```python
from build123d import *

# Parameters (mm, degrees)
ESQUISSE1_W       = 5.08
ESQUISSE1_H       = 2.54
EXTRUSION1_DEPTH  = 4
ESQUISSE2_R       = 0.915
EXTRUSION2_DEPTH  = 0.4
ESQUISSE3_R       = 0.535
EXTRUSION3_DEPTH  = 1.065
D_ME1_FACE_RADIUS = 0.535
D_ME1_HEIGHT      = 0.535
D_ME2_FACE_RADIUS = 0.535
D_ME2_HEIGHT      = 0.535


with BuildPart() as part:
    # Esquisse1 → Extrusion1 (new body)
    with BuildSketch(Plane.XY):
        with Locations((2.54, 1.27)):
            Rectangle(ESQUISSE1_W, ESQUISSE1_H)
    extrude(amount=EXTRUSION1_DEPTH)

    # Esquisse2 → Extrusion2 (add)
    with BuildSketch(Plane.XY.offset(4)):
        with Locations(Location((3.81, 1.27, 0), (0, 0, 180))):
            Circle(ESQUISSE2_R)
        with Locations(Location((1.27, 1.27, 0), (0, 0, 180))):
            Circle(ESQUISSE2_R)
    extrude(amount=EXTRUSION2_DEPTH)

    # Esquisse3 → Extrusion3 (add)
    with BuildSketch(Plane(origin=(0, 0, 0), x_dir=(-1, 0, 0), z_dir=(0, 0, -1))):
        with Locations((-3.81, 1.27)):
            Circle(ESQUISSE3_R)
        with Locations((-1.27, 1.27)):
            Circle(ESQUISSE3_R)
    extrude(amount=EXTRUSION3_DEPTH)

    # Dôme1: a dome of height H over a round flat face of radius A is a cap of a sphere of radius (A * A + H * H) / (2 * H)
    d_me1_r = (D_ME1_FACE_RADIUS * D_ME1_FACE_RADIUS + D_ME1_HEIGHT * D_ME1_HEIGHT) / (2 * D_ME1_HEIGHT)
    d_me1_base = Plane((3.81, 1.27, -1.065), z_dir=(0, 0, -1))
    with Locations(d_me1_base.offset(D_ME1_HEIGHT - d_me1_r)):
        d_me1_ball = Sphere(d_me1_r, mode=Mode.PRIVATE)
    add(split(d_me1_ball, bisect_by=d_me1_base, keep=Keep.TOP, mode=Mode.PRIVATE))

    # Dôme2: a dome of height H over a round flat face of radius A is a cap of a sphere of radius (A * A + H * H) / (2 * H)
    d_me2_r = (D_ME2_FACE_RADIUS * D_ME2_FACE_RADIUS + D_ME2_HEIGHT * D_ME2_HEIGHT) / (2 * D_ME2_HEIGHT)
    d_me2_base = Plane((1.27, 1.27, -1.065), z_dir=(0, 0, -1))
    with Locations(d_me2_base.offset(D_ME2_HEIGHT - d_me2_r)):
        d_me2_ball = Sphere(d_me2_r, mode=Mode.PRIVATE)
    add(split(d_me2_ball, bisect_by=d_me2_base, keep=Keep.TOP, mode=Mode.PRIVATE))


solid = part.part
```
CAD build for the part. Positions are in the model's coordinates, mm. A direction names the side the tool comes from. Round coordinates to 2 decimals unless told otherwise and drop trailing zeros. Write each loop counter-clockwise with the first axis right and the second up, starting at its lowest first coordinate (ties: lowest second). Pieces come first, ordered by that corner, then holes.
Item 1: Band-saw the part on D-D on x = 1.6. Write the cut outline in (y, z) (3 decimals), then the cut area to 3 significant figures.
Filled in:
outline: (0, 0) - (0.849, 0) - (0.849, -1.065) arc R0.421 ccw to (1.691, -1.065) - (1.691, 0) - (2.54, 0) - (2.54, 4) - (2.123, 4) - (2.123, 4.4) - (0.417, 4.4) - (0.417, 4) - (0, 4) - close
area: 12.0 mm2
Item 2: Tool access for faces 4 (the flat face through (0, 1, 2)), 5 (the flat face through (2.5, 1.3, 4)), 6 (the cylindrical face through (3.316, 1.065, -0.525)): list every direction of +Z, -Z, +X, -X, +Y, -Y with a clear straight run to the whole face (end or side of a thin tool).
Filled in:
face 4: +Z, -Z, -X, +Y, -Y
face 5: +Z
face 6: -Z
Item 3: Mould opens along X. For faces 1 (the flat face through (5.08, 1, 2)), 2 (the cylindrical face through (3.388, 2.082, 4.197)), 3 (the flat face through (3, 0, 2)) say: released by +X, released by -X, zero draft, split by the parting line, or undercut.
Filled in:
face 1: released by +X
face 2: undercut
face 3: zero draft
Item 4: Band-saw the part on C-C on y = 1.27. Write the cut outline in (x, z) (3 decimals), then the cut area to 3 significant figures.
Filled in:
outline: (0, 0) - (0.735, 0) - (0.735, -1.065) arc R0.535 ccw to (1.805, -1.065) - (1.805, 0) - (3.275, 0) - (3.275, -1.065) arc R0.535 ccw to (4.345, -1.065) - (4.345, 0) - (5.08, 0) - (5.08, 4) - (4.725, 4) - (4.725, 4.4) - (2.895, 4.4) - (2.895, 4) - (2.185, 4) - (2.185, 4.4) - (0.355, 4.4) - (0.355, 4) - (0, 4) - close
area: 25.0 mm2
Item 5: Drill centre lines: L1, parallel to Z at x = 2.8, y = 2.2; L2, parallel to Y at x = 1.3, z = -0.1; L3, parallel to Y at x = 3.75, z = -1.3. Where is each one in solid material? Low to high.
Filled in:
L1: z = 0 to 4
L2: y = 0.74 to 1.8
L3: y = 0.79 to 1.75
Item 6: Drop flat-ended pins along their axis: pin 1 Ø1.3 at (x, y) = (2.5, 1) entering from -Z; pin 2 Ø1 at (x, z) = (2, 3) entering from -Y. Give the stop position or say it passes through.
Filled in:
pin 1: stops at z = 0
pin 2: stops at y = 0
Item 7: Band-saw the part on A-A on x = 3.81. Write the cut outline in (y, z) (3 decimals).
Filled in:
outline: (0, 0) - (0.735, 0) - (0.735, -1.065) arc R0.535 ccw to (1.805, -1.065) - (1.805, 0) - (2.54, 0) - (2.54, 4) - (2.185, 4) - (2.185, 4.4) - (0.355, 4.4) - (0.355, 4) - (0, 4) - close
Item 8: Band-saw the part on B-B on z = -0.9. Write the cut outline in (x, y) (3 decimals).
Filled in:
outline: circle Ø1.07 at (1.27, 1.27); circle Ø1.07 at (3.81, 1.27)
